Geometry: final body of the model. Coordinates: model frame, mm. A direction names the side the tool comes from. Give positions to 0.01 mm unless a question says otherwise; leave off trailing zeros. Loops run counter-clockwise (first coordinate to the right, second up) from the corner with the lowest first, then second, coordinate; pieces in that order, holes last.
Autodesk Inventor part; units mm, degrees
ref_plane "YZ Plane" through (0, 0, 0) normal (1, 0, 0) x (0, 1, 0)
ref_plane "XZ Plane" through (0, 0, 0) normal (0, 1, 0) x (-1, 0, 0)
ref_plane "XY Plane" through (0, 0, 0) normal (0, 0, 1) x (1, 0, 0)
sketch "Skizze1" plane through (0, 0, 0) normal (0, 0, 1) x (1, 0, 0)
  line L0 (-3.6885, 36.0919) -> (-3.6885, -23.0081) construction
  arc A0 (-13.6885, -33.0081) -> (-3.6885, -23.0081) centre (-13.6885, -23.0081) ccw construction
  line L1 (-13.6885, -33.0081) -> (-72.7885, -33.0081) construction
  arc A1 (-82.7885, -23.0081) -> (-72.7885, -33.0081) centre (-72.7885, -23.0081) ccw construction
  line L2 (-82.7885, -23.0081) -> (-82.7885, 36.0919) construction
  arc A2 (-72.7885, 46.0919) -> (-82.7885, 36.0919) centre (-72.7885, 36.0919) ccw construction
  line L3 (-72.7885, 46.0919) -> (-13.6885, 46.0919) construction
  arc A3 (-3.6885, 36.0919) -> (-13.6885, 46.0919) centre (-13.6885, 36.0919) ccw construction
  arc A4 (-75.2885, 48.5919) -> (-85.2885, 38.5919) centre (-75.2885, 38.5919) ccw construction
  line L4 (-85.2885, 38.5919) -> (-85.2885, -25.5081) construction
  arc A5 (-85.2885, -25.5081) -> (-75.2885, -35.5081) centre (-75.2885, -25.5081) ccw construction
  line L5 (-75.2885, -35.5081) -> (-11.1885, -35.5081) construction
  arc A6 (-11.1885, -35.5081) -> (-1.1885, -25.5081) centre (-11.1885, -25.5081) ccw construction
  line L6 (-1.1885, -25.5081) -> (-1.1885, 38.5919) construction
  arc A7 (-1.1885, 38.5919) -> (-11.1885, 48.5919) centre (-11.1885, 38.5919) ccw construction
  line L7 (-11.1885, 48.5919) -> (-75.2885, 48.5919) construction
  line L8 (-13.6885, 45.9919) -> (-72.7885, 45.9919)
  arc A8 (-72.7885, 45.9919) -> (-82.6885, 36.0919) centre (-72.7885, 36.0919) ccw
  line L9 (-82.6885, 36.0919) -> (-82.6885, -23.0081)
  arc A9 (-82.6885, -23.0081) -> (-72.7885, -32.9081) centre (-72.7885, -23.0081) ccw
  line L10 (-72.7885, -32.9081) -> (-13.6885, -32.9081)
  arc A10 (-13.6885, -32.9081) -> (-3.7885, -23.0081) centre (-13.6885, -23.0081) ccw
  line L11 (-3.7885, -23.0081) -> (-3.7885, 36.0919)
  arc A11 (-3.7885, 36.0919) -> (-13.6885, 45.9919) centre (-13.6885, 36.0919) ccw
  line L12 (-47.3385, 46.0919) -> (-47.3385, 47.2919) construction
  line L13 (-47.3385, 47.2919) -> (-39.1385, 47.2919) construction
  line L14 (-39.1385, 46.0919) -> (-39.1385, 47.2919) construction
  line L15 (-68.3885, -33.0081) -> (-68.3885, -34.2081) construction
  line L16 (-63.1885, -33.0081) -> (-63.1885, -34.2081) construction
  line L17 (-63.1885, -34.2081) -> (-68.3885, -34.2081) construction
  line L18 (-23.2885, -33.0081) -> (-23.2885, -34.2081) construction
  line L19 (-18.0885, -34.2081) -> (-23.2885, -34.2081) construction
  line L20 (-18.0885, -33.0081) -> (-18.0885, -34.2081) construction
  line L21 (-68.0885, -32.9081) -> (-63.4885, -32.9081)
  line L22 (-63.4885, -32.9081) -> (-63.4885, -33.9081)
  line L23 (-63.4885, -33.9081) -> (-68.0885, -33.9081)
  line L24 (-68.0885, -33.9081) -> (-68.0885, -32.9081)
  line L25 (-22.9885, -32.9081) -> (-18.3885, -32.9081)
  line L26 (-18.3885, -32.9081) -> (-18.3885, -33.9081)
  line L27 (-18.3885, -33.9081) -> (-22.9885, -33.9081)
  line L28 (-22.9885, -33.9081) -> (-22.9885, -32.9081)
  line L29 (-47.0385, 45.9919) -> (-39.4385, 45.9919)
  line L30 (-39.4385, 45.9919) -> (-39.4385, 46.9919)
  line L31 (-39.4385, 46.9919) -> (-47.0385, 46.9919)
  line L32 (-47.0385, 46.9919) -> (-47.0385, 45.9919)
  line L33 (-62.0385, 43.9919) -> (-54.0385, 43.9919)
  line L34 (-54.0385, 43.9919) -> (-49.0385, 38.9919)
  line L35 (-49.0385, 38.9919) -> (-37.0385, 38.9919)
  line L36 (-37.0385, 38.9919) -> (-32.0385, 43.9919)
  line L37 (-32.0385, 43.9919) -> (-24.0385, 43.9919)
  line L38 (-24.0385, 43.9919) -> (-24.0385, 37.4919)
  line L39 (-24.0385, 37.4919) -> (-62.0385, 37.4919)
  line L40 (-62.0385, 37.4919) -> (-62.0385, 43.9919)
  line L41 (-48.0385, 43.9919) -> (-38.0385, 43.9919)
  line L42 (-38.0385, 43.9919) -> (-38.0385, 40.9919)
  line L43 (-38.0385, 40.9919) -> (-48.0385, 40.9919)
  line L44 (-48.0385, 40.9919) -> (-48.0385, 43.9919)
  circle A12 centre (-74.3885, -23.6081) radius 4.075 construction
  circle A13 centre (-12.0885, 36.6919) radius 4.075 construction
  circle A14 centre (-12.0885, 36.6919) radius 5.075
  circle A15 centre (-74.3885, -23.6081) radius 5.075
  arc A16 (-56.277, -27.2081) -> (-60.2001, -27.2081) centre (-58.2385, -25.6581) ccw construction
  arc A17 (-26.277, -27.2081) -> (-30.2001, -27.2081) centre (-28.2385, -25.6581) ccw construction
  arc A18 (-60.1167, 40.3919) -> (-56.3604, 40.3919) centre (-58.2385, 38.7419) ccw construction
  arc A19 (-30.1167, 40.3919) -> (-26.3604, 40.3919) centre (-28.2385, 38.7419) ccw construction
  circle A20 centre (-58.2385, 38.7419) radius 3
  circle A21 centre (-28.2385, 38.7419) radius 3
  circle A22 centre (-58.2385, -25.6581) radius 3
  circle A23 centre (-28.2385, -25.6581) radius 3
  point P0 (0, 0)
  dimension "d0" = 0.1
  dimension "d1" = 0.3
  dimension "d2" = 0.3
  dimension "d3" = 0.3
  dimension "d4" = 0.3
  dimension "d5" = 0.3
  dimension "d6" = 0.3
  dimension "d7" = 0.3
  dimension "d8" = 0.3
  dimension "d9" = 0.3
  dimension "d10" = 135
  dimension "d11" = 1.5
  dimension "d12" = 2
  dimension "d13" = 8
  dimension "d14" = 8
  dimension "d15" = 12
  dimension "d17" = 2
  dimension "d18" = 10
  dimension "d19" = 1
  dimension "d20" = 2
  dimension "d21" = 3
  dimension "d22" = 2
  dimension "d25" = 1
  dimension "d26" = 1
  dimension "d28" = 6
  dimension "d29" = 6
  dimension "d30" = 6
  dimension "d31" = 6
extrude "Extrusion1" add sketch "Skizze1" along normal blind 0.8
fillet "Rundung1" radius 1 12 edges at (-48.0385, 43.9919, 0.4) (-48.0385, 40.9919, 0.4) (-38.0385, 40.9919, 0.4) (-38.0385, 43.9919, 0.4) (-54.0385, 43.9919, 0.4) (-49.0385, 38.9919, 0.4) (-37.0385, 38.9919, 0.4) (-32.0385, 43.9919, 0.4) (-24.0385, 43.9919, 0.4) (-24.0385, 37.4919, 0.4) (-62.0385, 37.4919, 0.4) (-62.0385, 43.9919, 0.4)
equation "\"d1\" = d4"
equation "\"d2\" = d1"
equation "\"d3\" = d1"
equation "\"d5\" = d4"
equation "\"d6\" = d4"
equation "\"d7\" = d9"
equation "\"d8\" = d7"
equation "\"d9\" = d4"
equation "\"d26\" = d25"
equation "\"d29\" = d28"
equation "\"d30\" = d28"
equation "\"d31\" = d28"
properties part number "Boden"
Q1. Section query B-B, the plane x = -52.5. Return loops of the section in (y, z), and give its area (3 significant figures).
Q2. Material intervals for probe 1 along Y at (x, z) = (-42.5, 0.4); probe 2 along Y at (x, z) = (-61, 0.45); probe 3 along X at (y, z) = (42, 0.35), sorted ascending.
Q3. Mould query, pull axis Y, two halves, no side actions, for faces 3 (the face through (-44, 7, 0.8)), 4 (the face through (-6.61, -29.93, 0.39)), 5 (the face through (-31.236, -25.79, 0.394)), 6 (the face through (-79.87, 43.01, 0.39)). Classes: +Y half, -Y half, draft (parallel to the pull), parting line (faces both ways), or undercut.
Q4. Section query C-C, the plane z = 0.55. State how many separate pieces and enclosed holes the cut face has, and give its area (3 significant figures).
Q5. Section query D-D, the plane x = -15.5. Return loops of the section in (y, z).
Q6. Section query A-A, the plane x = -42.5. Return loops of the section in (y, z).
Q7. Reachability of faces 1 (the face through (-6.8, 43.2, 0.4)), 2 (the face through (-34.57, 41.46, 0.39)) from +Z, -Z, +X, -X, +Y, -Y: full face, straight path, thin tool, end or side. Return the list, or none.
Resolved:
1. outline: (-32.91, 0) - (37.49, 0) - (37.49, 0.8) - (-32.91, 0.8) - close; (42.45, 0) - (45.99, 0) - (45.99, 0.8) - (42.45, 0.8) - close
1. area: 59.2 mm2
2. probe 1: y = -32.91 to 37.49, 38.99 to 40.99, 43.99 to 46.99
2. probe 2: y = -32.91 to -26.83, -24.49 to 37.49, 43.99 to 45.99
2. probe 3: x = -80.73 to -62.04, -52.05 to -48.04, -38.04 to -34.03, -24.04 to -5.74
3. face 3: draft
3. face 4: -Y half
3. face 5: undercut
3. face 6: +Y half
4. separate pieces: 1
4. enclosed holes: 6
4. area: 5,740 mm2
5. outline: (-32.91, 0) - (32.93, 0) - (32.93, 0.8) - (-32.91, 0.8) - close; (40.45, 0) - (45.99, 0) - (45.99, 0.8) - (40.45, 0.8) - close
6. outline: (-32.91, 0) - (37.49, 0) - (37.49, 0.8) - (-32.91, 0.8) - close; (38.99, 0) - (40.99, 0) - (40.99, 0.8) - (38.99, 0.8) - close; (43.99, 0) - (46.99, 0) - (46.99, 0.8) - (43.99, 0.8) - close
7. face 1: +Z, -Z, +X, +Y
7. face 2: +Z, -Z
